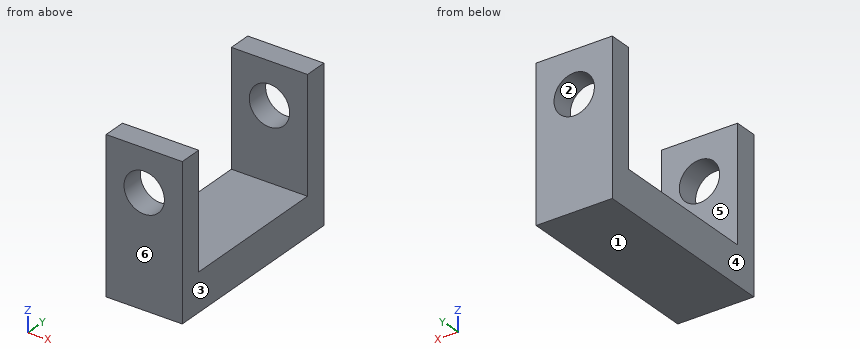
```python
from build123d import *

# Parameters (mm, degrees)
SKETCH2_W           = 26
SKETCH2_H           = 10
BOSS_EXTRUDE1_DEPTH = 20
SKETCH3_W           = 10
SKETCH3_H           = 20
CUT_EXTRUDE1_DEPTH  = 15
SKETCH4_R           = 2.65
CUT_EXTRUDE2_DEPTH  = 34.181320046


with BuildPart() as part:
    # Sketch2 → Boss-Extrude1 (new body)
    with BuildSketch(Plane(origin=(0, 0, 0), x_dir=(0, 1, 0), z_dir=(0, 0, 1))):
        Rectangle(SKETCH2_W, SKETCH2_H)
    extrude(amount=BOSS_EXTRUDE1_DEPTH)

    # Sketch3 → Cut-Extrude1 (cut)
    with BuildSketch(Plane.XY.offset(20)):
        Rectangle(SKETCH3_W, SKETCH3_H)
    extrude(amount=-CUT_EXTRUDE1_DEPTH, mode=Mode.SUBTRACT)

    # Sketch4 → Cut-Extrude2 (cut, through all)
    with BuildSketch(Plane.XZ.offset(13)):
        with Locations(Location((0, 14.5, 0), (0, 0, 270))):
            Circle(SKETCH4_R)
    extrude(amount=-CUT_EXTRUDE2_DEPTH, mode=Mode.SUBTRACT)


solid = part.part
```
Check sheet for the modelled part. Datum: model origin and axes. Units: mm. Face numbers are marked on the shaded views. A direction names the side the tool comes from. Round coordinates to 2 decimals unless told otherwise and drop trailing zeros. Order: outer loops, then holes, each group sorted by start corner. A loop starts at its lowest first (then second) coordinate and runs counter-clockwise, first axis right, second up.
1) Section check A-A (z = 14.5). Record the boundary of the cut face in (x, y), and give its area (3 significant figures).
2) Go/stop test with flat-tipped pins: pin 1 Ø2 at (x, y) = (-1, -1) entering from +Z; pin 2 Ø4 at (x, z) = (0, 14.5) entering from +Y. Record where each tip stops, or that it passes through.
3) Section check D-D (x = 4). Record the boundary of the cut face in (y, z), and give its area (3 significant figures).
4) Mould release check, pull along X, two halves, no side actions. Record for the marked faces 1, 2, 3 and 4: +X half, -X half, draft (parallel to the pull), parting line (faces both ways), or undercut.
5) Section check B-B (x = 0). Record the boundary of the cut face in (y, z), and give its area (3 significant figures).
6) Scan lines: line 1 (X direction, y = 12.25, z = 14.5); line 2 (Y direction, x = 3.5, z = 19); line 3 (Z direction, x = 4.25, y = 8.5). Record each from-to range of solid material in increasing order.
7) Tool access check on the marked faces 5 and 6. Record the directions out of +Z, -Z, +X, -X, +Y, -Y that give a thin tool (end or side, any length) a straight path to the whole face; none if there is none.
8) Section check C-C (z = 10.5). Record the boundary of the cut face in (x, y).
Result:
1. outline: (-5, -13) - (-2.65, -13) - (-2.65, -10) - (-5, -10) - close; (-5, 10) - (-2.65, 10) - (-2.65, 13) - (-5, 13) - close; (2.65, -13) - (5, -13) - (5, -10) - (2.65, -10) - close; (2.65, 10) - (5, 10) - (5, 13) - (2.65, 13) - close
1. area: 28.2 mm2
2. pin 1: stops at z = 5
2. pin 2: passes through
3. outline: (-13, 0) - (13, 0) - (13, 20) - (10, 20) - (10, 5) - (-10, 5) - (-10, 20) - (-13, 20) - close
3. area: 220 mm2
4. face 1: draft
4. face 2: undercut
4. face 3: +X half
4. face 4: -X half
5. outline: (-13, 0) - (13, 0) - (13, 11.85) - (10, 11.85) - (10, 5) - (-10, 5) - (-10, 11.85) - (-13, 11.85) - close; (-13, 17.15) - (-10, 17.15) - (-10, 20) - (-13, 20) - close; (10, 17.15) - (13, 17.15) - (13, 20) - (10, 20) - close
5. area: 188 mm2
6. line 1: x = -5 to -2.65, 2.65 to 5
6. line 2: y = -13 to -10, 10 to 13
6. line 3: z = 0 to 5
7. face 5: +Z, +X, -X
7. face 6: +Z, -Z, +X, -X, -Y
8. outline: (-5, -13) - (5, -13) - (5, -10) - (-5, -10) - close; (-5, 10) - (5, 10) - (5, 13) - (-5, 13) - close
